Geometry check sheet. Reference: the model listing, model coordinates, mm. Face numbers are marked on the shaded views. A direction names the side the tool comes from. Coordinates: 2 decimals unless noted, no trailing zeros. Write each loop counter-clockwise with the first axis right and the second up, starting at its lowest first coordinate (ties: lowest second). Pieces come first, ordered by that corner, then holes. Notation, with made-up numbers: (0.25, -34.75) -> (19.25, -34.75) arc R11 ccw to (19.25, -19.75) -> close; hole circle Ø8 at (18.5, 6.5). An arc over 180 degrees is marked (long way). Use a Markdown table: item, result.
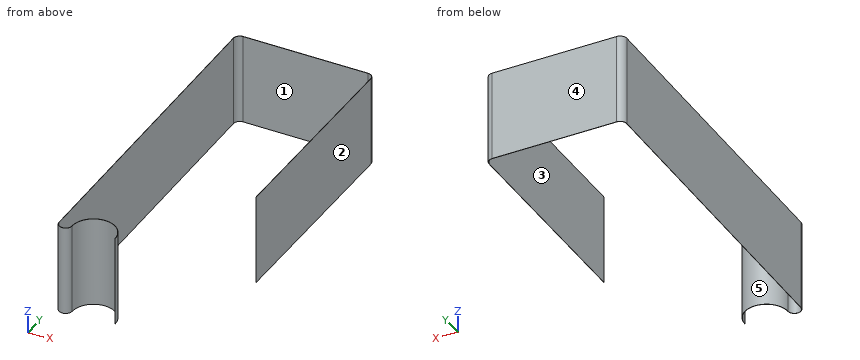
```python
from build123d import *

# Parameters (mm, degrees)
SKETCH2_W = 0.5
SKETCH2_H = 210


with BuildPart() as part:
    # Sweep1: sweep along a path in Sketch1
    with BuildLine(Plane.XY) as sweep1_path:
        Line((5, 1131.07306524), (5, 1631.07306524))
        ThreePointArc((5, 1631.07306524), (0.606601718, 1641.679666958), (-10, 1646.07306524))
        Line((-10, 1646.07306524), (-300, 1646.07306524))
        ThreePointArc((-300, 1646.07306524), (-310.657609176, 1641.628413015), (-314.99930284, 1630.928447459))
        Line((-314.99930284, 1630.928447459), (-307.545742915, 857.868578543))
        ThreePointArc((-307.545742915, 857.868578543), (-292.474130344, 843.013370614), (-277.546440075, 858.013196323))
        ThreePointArc((-277.546440075, 858.013196323), (-227.546440075, 908.013196323), (-177.546440075, 858.013196323))
    # Sketch2 → Sweep1 (sweep)
    with BuildSketch(Plane(origin=(0, 1131.07306524, 0), x_dir=(1, 0, 0), z_dir=(0, 1, 0))):
        with Locations((5, 0)):
            Rectangle(SKETCH2_W, SKETCH2_H)
    sweep(path=sweep1_path.line)


solid = part.part
```
Item 1: Section check D-D on x = -104. Record the boundary of the cut face in (y, z).
Answer block:
| item | result |
|---|---|
| outline | (1645.82, -105) -> (1646.32, -105) -> (1646.32, 105) -> (1645.82, 105) -> close |
Item 2: Depth check by flat-ended pin: P1, Ø2, axis at x = -252.5, z = 37.5, coming from the -Y side; P2, Ø1, axis at x = -41.5, z = -35.5, coming from the -Y side; P3, Ø3, axis at x = -253.5, z = 56.5, coming from the -Y side. Enter the tip coordinate at first touch or a pass-through.
Answer block:
| item | result |
|---|---|
| P1 | stops at y = 900.46 |
| P2 | stops at y = 1645.82 |
| P3 | stops at y = 899.5 |
Item 3: Thickness scan on L1, parallel to X at y = 1413, z = 59.5; L2, parallel to X at y = 1383, z = 17.5; L3, parallel to Y at x = -228, z = 75. Record the ranges inside material, lowest first. Write a range as [from, to].
Answer block:
| item | result |
|---|---|
| L1 | x = [-313.15, -312.65], [4.75, 5.25] |
| L2 | x = [-312.86, -312.36], [4.75, 5.25] |
| L3 | y = [907.76, 908.26], [1645.82, 1646.32] |
Item 4: Section check C-C on z = 29.5. Record the boundary of the cut face in (x, y), then the cut area to 3 significant figures.
Answer block:
| item | result |
|---|---|
| outline | (-315.25, 1630.93) -> (-307.8, 857.87) arc R15.25 ccw to (-277.3, 858.01) arc R49.75 cw to (-177.8, 858.01) -> (-177.3, 858.01) arc R50.25 ccw to (-277.8, 858.01) arc R14.75 cw to (-307.3, 857.87) -> (-314.75, 1630.93) arc R14.75 cw to (-300, 1645.82) -> (-10, 1645.82) arc R14.75 cw to (4.75, 1631.07) -> (4.75, 1131.07) -> (5.25, 1131.07) -> (5.25, 1631.07) arc R15.25 ccw to (-10, 1646.32) -> (-300, 1646.32) arc R15.25 ccw to start |
| area | 907 mm^2 |
Item 5: Mould release check, pull along Y, two halves, no side actions. Record for the marked faces 3, 4 and 5: +Y half, -Y half, draft (parallel to the pull), parting line (faces both ways), or undercut.
Answer block:
| item | result |
|---|---|
| face 3 | draft |
| face 4 | +Y half |
| face 5 | undercut |
Item 6: Tool access check on the marked faces 1 and 2. Record the directions out of +Z, -Z, +X, -X, +Y, -Y that give a thin tool (end or side, any length) a straight path to the whole face; none if there is none.
Answer block:
| item | result |
|---|---|
| face 1 | +Z, -Z |
| face 2 | +Z, -Z, +X, +Y, -Y |
Item 7: Section check B-B on y = 1385.5. Record the boundary of the cut face in (x, z), then the cut area to 3 significant figures.
Answer block:
| item | result |
|---|---|
| outline | (-312.88, -105) -> (-312.38, -105) -> (-312.38, 105) -> (-312.88, 105) -> close; (4.75, -105) -> (5.25, -105) -> (5.25, 105) -> (4.75, 105) -> close |
| area | 210 mm^2 |
Item 8: Section check A-A on x = -286. Record the boundary of the cut face in (y, z).
Answer block:
| item | result |
|---|---|
| outline | (844.24, -105) -> (844.8, -105) -> (844.8, 105) -> (844.24, 105) -> close; (1645.82, -105) -> (1646.32, -105) -> (1646.32, 105) -> (1645.82, 105) -> close |
